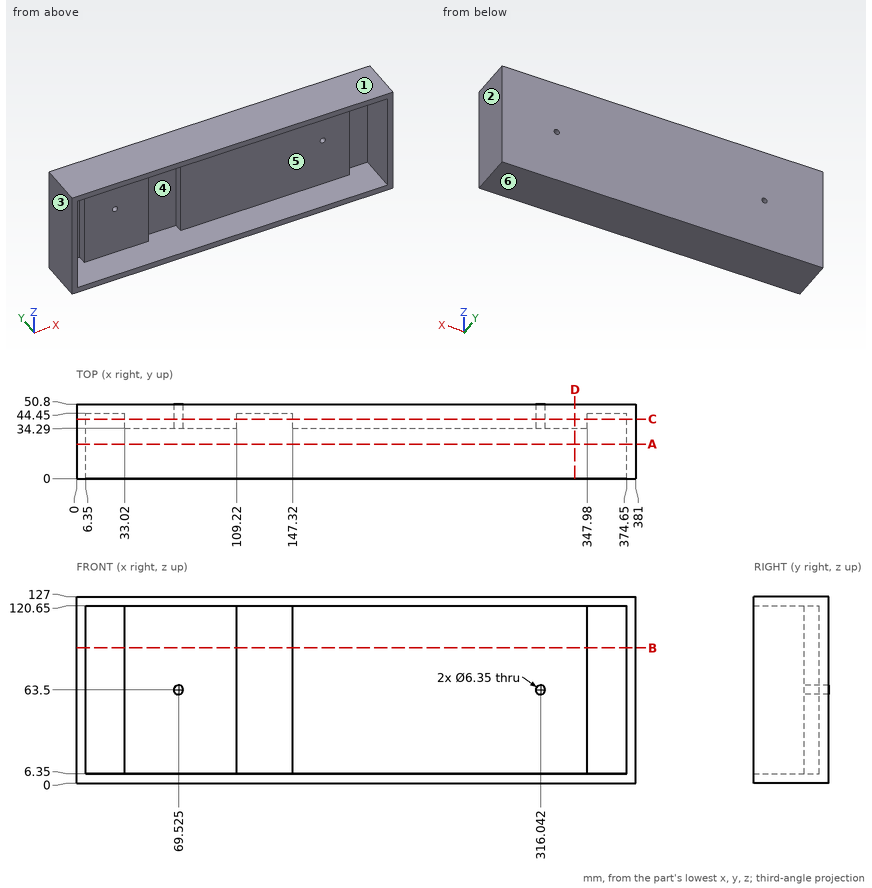
Job drawing, mm, ordinate dimensions from the low corner. One solid piece. A direction names the side the tool comes from. Coordinates: 2 decimals unless noted, no trailing zeros. Write each loop counter-clockwise with the first axis right and the second up, starting at its lowest first coordinate (ties: lowest second). Pieces come first, ordered by that corner, then holes.
Item 1: Probe line 1 (X direction, y = 46, z = 63); line 2 (Z direction, x = 196.5, y = 4); line 3 (X direction, y = 32.5, z = 50). List the from-to ranges inside material, lowest first.
Item 2: Slice it at C-C (y = 40.5). Count the separate pieces of the cut face and the enclosed holes in it, and give its area (3 significant figures).
Item 3: Pin check, flat tips, straight feed: pin 1 (13.5 mm diameter, centred on y = 26, z = 40, fed in from -X); pin 2 (5 mm diameter, centred on x = 69.52, z = 63.5, fed in from -Y); pin 3 (23 mm diameter, centred on x = 88.5, z = 78, fed in from -Y); pin 4 (8 mm diameter, centred on x = 21, z = 90, fed in from -Y). Stop position of each tip, or through.
Item 4: Which spindle directions (+Z, -Z, +X, -X, +Y, -Y) get a long thin tool onto all of the face, cutting with end or side? Do the marked faces 5 and 6. Say none if no direction does.
Item 5: Slice it at A-A (y = 23.5). Write the cut outline in (x, z), and give its area (3 significant figures).
Item 6: Mould opens along X. For the marked faces 1, 2, 3 and 4 say: released by +X, released by -X, zero draft, split by the parting line, or undercut.
Item 7: Slice it at B-B (z = 92). Write the cut outline in (x, y), and give its area (3 significant figures).
Item 8: Slice it at D-D (x = 339.5). Write the cut outline in (y, z), and give its area (3 significant figures).
Results found:
1. line 1: x = 0 to 66.39, 72.66 to 312.91, 319.18 to 381
1. line 2: z = 0 to 6.35, 120.65 to 127
1. line 3: x = 0 to 6.35, 374.65 to 381
2. separate pieces: 1
2. enclosed holes: 5
2. area: 37,900 mm2
3. pin 1: stops at x = 0
3. pin 2: passes through
3. pin 3: stops at y = 34.29
3. pin 4: stops at y = 44.45
4. face 5: -Y
4. face 6: -Z, +X, -X, +Y, -Y
5. outline: (0, 0) - (381, 0) - (381, 127) - (0, 127) - close; hole (6.35, 6.35) - (374.65, 6.35) - (374.65, 120.65) - (6.35, 120.65) - close
5. area: 6,290 mm2
6. face 1: zero draft
6. face 2: released by +X
6. face 3: released by -X
6. face 4: undercut
7. outline: (0, 0) - (6.35, 0) - (6.35, 44.45) - (33.02, 44.45) - (33.02, 34.29) - (109.22, 34.29) - (109.22, 44.45) - (147.32, 44.45) - (147.32, 34.29) - (347.98, 34.29) - (347.98, 44.45) - (374.65, 44.45) - (374.65, 0) - (381, 0) - (381, 50.8) - (0, 50.8) - close
7. area: 5,800 mm2
8. outline: (0, 0) - (50.8, 0) - (50.8, 127) - (0, 127) - (0, 120.65) - (34.29, 120.65) - (34.29, 6.35) - (0, 6.35) - close
8. area: 2,530 mm2
